```python
from build123d import *

# Parameters (mm, degrees)
F2_DEPTH = 3
F3_DEPTH = 10
F4_R     = 2
F6_DEPTH = 4.4


with BuildPart() as f2:
    # F1 (on Top) → F2 (new body)
    with BuildSketch(Plane.XY):
        with BuildLine():
            Line((45.8, 50.8), (-45.8, 50.8))
            ThreePointArc((-45.8, 50.8), (-49.3355339059, 49.3355339059), (-50.8, 45.8))
            Line((-50.8, 45.8), (-50.8, -45.8))
            ThreePointArc((-50.8, -45.8), (-49.3355339059, -49.3355339059), (-45.8, -50.8))
            Line((-45.8, -50.8), (45.8, -50.8))
            ThreePointArc((45.8, -50.8), (49.3355339059, -49.3355339059), (50.8, -45.8))
            Line((50.8, -45.8), (50.8, 45.8))
            ThreePointArc((50.8, 45.8), (49.3355339059, 49.3355339059), (45.8, 50.8))
        make_face()
        with BuildLine():
            ThreePointArc((-48, 43), (-46.5355339059, 46.5355339059), (-43, 48))
            Line((-43, 48), (43, 48))
            ThreePointArc((43, 48), (46.5355339059, 46.5355339059), (48, 43))
            Line((48, 43), (48, -43))
            ThreePointArc((48, -43), (46.5355339059, -46.5355339059), (43, -48))
            Line((43, -48), (-43, -48))
            ThreePointArc((-43, -48), (-46.5355339059, -46.5355339059), (-48, -43))
            Line((-48, -43), (-48, 43))
        make_face(mode=Mode.SUBTRACT)
        with BuildLine():
            Line((43, 48), (-43, 48))
            ThreePointArc((-43, 48), (-46.5355339059, 46.5355339059), (-48, 43))
            Line((-48, 43), (-48, -43))
            ThreePointArc((-48, -43), (-46.5355339059, -46.5355339059), (-43, -48))
            Line((-43, -48), (43, -48))
            ThreePointArc((43, -48), (46.5355339059, -46.5355339059), (48, -43))
            Line((48, -43), (48, 43))
            ThreePointArc((48, 43), (46.5355339059, 46.5355339059), (43, 48))
        make_face()
        Polygon((45, -42.8786796564), (45, -45), (42.8786796564, -45), (-42.8786796564, -45), (-45, -45), (-45, -42.8786796564), (-45, 42.8786796564), (-45, 45), (-42.8786796564, 45), (42.8786796564, 45), (45, 45), (45, 42.8786796564), align=None, mode=Mode.SUBTRACT)
        Polygon((-45, 42.8786796564), (-45, -42.8786796564), (-2.1213203436, 0), align=None)
        Polygon((0, 2.1213203436), (42.8786796564, 45), (-42.8786796564, 45), align=None)
        Polygon((2.1213203436, 0), (45, -42.8786796564), (45, 42.8786796564), align=None)
        Polygon((-42.8786796564, -45), (42.8786796564, -45), (0, -2.1213203436), align=None)
        Polygon((42.8786796564, -45), (45, -45), (45, -42.8786796564), (2.1213203436, 0), (45, 42.8786796564), (45, 45), (42.8786796564, 45), (0, 2.1213203436), (-42.8786796564, 45), (-45, 45), (-45, 42.8786796564), (-2.1213203436, 0), (-45, -42.8786796564), (-45, -45), (-42.8786796564, -45), (0, -2.1213203436), align=None)
    extrude(amount=-F2_DEPTH)

    # F1 (on Top) → F3 (join)
    with BuildSketch(Plane.XY):
        with BuildLine():
            Line((43, 48), (-43, 48))
            ThreePointArc((-43, 48), (-46.5355339059, 46.5355339059), (-48, 43))
            Line((-48, 43), (-48, -43))
            ThreePointArc((-48, -43), (-46.5355339059, -46.5355339059), (-43, -48))
            Line((-43, -48), (43, -48))
            ThreePointArc((43, -48), (46.5355339059, -46.5355339059), (48, -43))
            Line((48, -43), (48, 43))
            ThreePointArc((48, 43), (46.5355339059, 46.5355339059), (43, 48))
        make_face()
        Polygon((45, -42.8786796564), (45, -45), (42.8786796564, -45), (-42.8786796564, -45), (-45, -45), (-45, -42.8786796564), (-45, 42.8786796564), (-45, 45), (-42.8786796564, 45), (42.8786796564, 45), (45, 45), (45, 42.8786796564), align=None, mode=Mode.SUBTRACT)
        Polygon((42.8786796564, -45), (45, -45), (45, -42.8786796564), (2.1213203436, 0), (45, 42.8786796564), (45, 45), (42.8786796564, 45), (0, 2.1213203436), (-42.8786796564, 45), (-45, 45), (-45, 42.8786796564), (-2.1213203436, 0), (-45, -42.8786796564), (-45, -45), (-42.8786796564, -45), (0, -2.1213203436), align=None)
    extrude(amount=F3_DEPTH)

    # F4
    f4_edges = [f2.edges().sort_by_distance(p)[0] for p in [
        (0, 50.8, -3),
        (-49.335534, 49.335534, -3),
        (-50.8, 0, -3),
        (-49.335534, -49.335534, -3),
        (0, -50.8, -3),
        (49.335534, -49.335534, -3),
        (50.8, 0, -3),
        (49.335534, 49.335534, -3),
    ]]
    fillet(f4_edges, radius=F4_R)

    # F5 (on face) → F6 (cut)
    with BuildSketch(Plane(origin=(0, 0, -3), x_dir=(1, 0, 0), z_dir=(0, 0, -1))):
        Polygon((20.75, 37.8), (-20.75, 37.8), (-19, 27.2), (19, 27.2), align=None)
    extrude(amount=-F6_DEPTH, mode=Mode.SUBTRACT)


solid = f2.part
```
The listing builds one solid part. Answer for the finished solid, in the listing's coordinates (mm). A direction names the side the tool comes from. Give positions to 0.01 mm unless a question says otherwise; leave off trailing zeros. Order: outer loops, then holes, each group sorted by start corner. A loop starts at its lowest first (then second) coordinate and runs counter-clockwise, first axis right, second up. Notation, with made-up numbers: (-22.5, -25.5) -> (7.5, -25.5) arc R28 ccw to (7.5, 13.5) -> close; hole circle Ø3 at (-14, 2). An arc over 180 degrees is marked (long way). Answer as a JSON object with one key per item and string values. Group by question number.
Item 1: The part is cut by section C-C on y = -28.5. Write down the section's boundary in (x, z).
Item 2: Determine the mould class of faces 1 (the flat face through (-48, 1, 5)), 2 (the flat face through (0, 0, 10)), 3 (the flat face through (-1, 29, 0)) for opening direction X: pulls with the +X half, pulls with the -X half, needs draft (parallel to the pull), parting line crosses it, or undercut.
Item 3: Flat-ended cylindrical pins translate along their axes: pin 1 (3 mm diameter, centred on y = -0.5, z = 6, fed in from +X); pin 2 (5 mm diameter, centred on x = -7.5, z = 4, fed in from +Y); pin 3 (1 mm diameter, centred on x = -5.5, y = 12.5, fed in from +Z). Find the tip coordinate at first contact, or state that the pin passes through.
Item 4: A tool of negligible diameter and unlimited length cuts with its end or side. For faces 4 (the cylindrical face through (46, -47, 5)), 5 (the flat face through (-21.74, -23.86, 4.93)), 6 (the flat face through (48, -1, 5)), 7 (the flat face through (0, -37.8, -2)), 8 (the cylindrical face through (47, 46, 5)), from which of +Z, -Z, +X, -X, +Y, -Y can it reach the whole face along a straight path? Write none if from no direction.
Item 5: The part is cut by section A-A on z = 3.5. Write down the section's boundary in (x, y), and give its area (3 significant figures).
Item 6: Consider L1, parallel to X at y = -11.5, z = 0.5; L2, parallel to X at y = 12.5, z = 8; L3, parallel to Y at x = -30, z = 6. Determine where each line is inside the solid, lowest interval first. Write a range as from..to.
Item 7: The part is cut by section B-B on x = -10.5. Write down the section's boundary in (y, z), and give its area (3 significant figures).
Item 8: The part is cut by section D-D on x = 26.5. Write down the section's boundary in (y, z).
Result set:
{
 "1": {"outline": "(-50.8, -1) arc R2 ccw to (-48.8, -3) -> (-19.21, -3) -> (-19.21, 0) -> (-26.38, 0) -> (-26.38, 10) -> (-30.62, 10) -> (-30.62, 0) -> (-45, 0) -> (-45, 10) -> (-48, 10) -> (-48, 0) -> (-50.8, 0) -> close; (19.21, -3) -> (48.8, -3) arc R2 ccw to (50.8, -1) -> (50.8, 0) -> (48, 0) -> (48, 10) -> (45, 10) -> (45, 0) -> (30.62, 0) -> (30.62, 10) -> (26.38, 10) -> (26.38, 0) -> (19.21, 0) -> close"},
 "2": {"face 1": "pulls with the -X half", "face 2": "needs draft", "face 3": "undercut"},
 "3": {"pin 1": "x = 48", "pin 2": "y = 48", "pin 3": "z = 0"},
 "4": {"face 4": "+Z, +X, -Y", "face 5": "+Z", "face 6": "+Z, +X, +Y, -Y", "face 7": "+Z, -Z", "face 8": "+Z, +X, +Y"},
 "5": {"outline": "(-48, -43) arc R5 ccw to (-43, -48) -> (43, -48) arc R5 ccw to (48, -43) -> (48, 43) arc R5 ccw to (43, 48) -> (-43, 48) arc R5 ccw to (-48, 43) -> close; hole (-45, -42.88) -> (-2.12, 0) -> (-45, 42.88) -> close; hole (-42.88, -45) -> (42.88, -45) -> (0, -2.12) -> close; hole (-42.88, 45) -> (0, 2.12) -> (42.88, 45) -> close; hole (2.12, 0) -> (45, -42.88) -> (45, 42.88) -> close", "area": "1,840 mm²"},
 "6": {"L1": "-48..-45, -13.62..-9.38, 9.38..13.62, 45..48", "L2": "-48..-45, -14.62..-10.38, 10.38..14.62, 45..48", "L3": "-48..-45, -32.12..-27.88, 27.88..32.12, 45..48"},
 "7": {"outline": "(-50.8, -1) arc R2 ccw to (-48.8, -3) -> (-37.8, -3) -> (-37.8, 0) -> (-45, 0) -> (-45, 10) -> (-48, 10) -> (-48, 0) -> (-50.8, 0) -> close; (-27.2, -3) -> (48.8, -3) arc R2 ccw to (50.8, -1) -> (50.8, 0) -> (48, 0) -> (48, 10) -> (45, 10) -> (45, 0) -> (12.62, 0) -> (12.62, 10) -> (8.38, 10) -> (8.38, 0) -> (-8.38, 0) -> (-8.38, 10) -> (-12.62, 10) -> (-12.62, 0) -> (-27.2, 0) -> close", "area": "416 mm²"},
 "8": {"outline": "(-50.8, -1) arc R2 ccw to (-48.8, -3) -> (48.8, -3) arc R2 ccw to (50.8, -1) -> (50.8, 0) -> (48, 0) -> (48, 10) -> (45, 10) -> (45, 0) -> (28.62, 0) -> (28.62, 10) -> (24.38, 10) -> (24.38, 0) -> (-24.38, 0) -> (-24.38, 10) -> (-28.62, 10) -> (-28.62, 0) -> (-45, 0) -> (-45, 10) -> (-48, 10) -> (-48, 0) -> (-50.8, 0) -> close"}
}
